Build history of the part. All positions in model axes, mm. A direction names the side the tool comes from. Round coordinates to 2 decimals unless told otherwise and drop trailing zeros. Loops run counter-clockwise (first coordinate to the right, second up) from the corner with the lowest first, then second, coordinate; pieces in that order, holes last. Notation, with made-up numbers: (23, 76) - (36, 76) arc R25 cw to (36, 95) - close; hole circle Ø4 at (-19, 89). An arc over 180 degrees is marked (long way). Put each result on its own line as item: value. Start each with the question number.
from build123d import *

# Parameters (mm, degrees)
SKETCH1_R               = 3.9
BOSS_EXTRUDE1_DEPTH     = 7
SKETCH2_R               = 6
BOSS_EXTRUDE2_DEPTH     = 1
SKETCH3_R               = 9.9
BOSS_EXTRUDE3_DEPTH     = 7
BOSS_EXTRUDE4_DEPTH     = 1
SKETCH5_R               = 1.6
CUT_EXTRUDE1_DEPTH      = 20.300518128
CUT_EXTRUDE2_DEPTH      = 20.300518128
CUT_EXTRUDE2_DEPTH_BACK = 5
SKETCH7_R               = 3.5
CHAMFER1_SIZE           = 1


with BuildPart() as part:
    # Sketch1 → Boss-Extrude1 (new body)
    with BuildSketch(Plane(origin=(0, 0, 0), x_dir=(1, 0, 0), z_dir=(0, 1, 0))):
        with Locations(Location((0, 0, 0), (0, 0, 270))):
            Circle(SKETCH1_R)
    extrude(amount=BOSS_EXTRUDE1_DEPTH)

    # Sketch2 → Boss-Extrude2 (add)
    with BuildSketch(Plane(origin=(0, 0, 0), x_dir=(-1, 0, 0), z_dir=(0, -1, 0))):
        with Locations(Location((0, 0, 0), (0, 0, 90))):
            Circle(SKETCH2_R)
    extrude(amount=BOSS_EXTRUDE2_DEPTH)

    # Sketch3 → Boss-Extrude3 (add)
    with BuildSketch(Plane(origin=(0, -1, 0), x_dir=(-1, 0, 0), z_dir=(0, -1, 0))):
        with Locations(Location((0, 2.5, 0), (0, 0, 90))):
            Circle(SKETCH3_R)
    extrude(amount=BOSS_EXTRUDE3_DEPTH)

    # Sketch4 → Boss-Extrude4 (add)
    with BuildSketch(Plane(origin=(0, -8, 0), x_dir=(-1, 0, 0), z_dir=(0, -1, 0))):
        with BuildLine():
            ThreePointArc((-11.736694594, 0), (0, -9.5), (11.736694594, 0))
            ThreePointArc((11.736694594, 0), (0, 9.5), (-11.736694594, 0))
        make_face()
    extrude(amount=BOSS_EXTRUDE4_DEPTH)

    # Sketch5 → Cut-Extrude1 (cut, through all)
    with BuildSketch(Plane(origin=(0, 0, 0), x_dir=(1, 0, 0), z_dir=(0, 1, 0))):
        with Locations(Location((5.5, 0, 0), (0, 0, 270))):
            Circle(SKETCH5_R)
        with Locations(Location((-5.5, 0, 0), (0, 0, 270))):
            Circle(SKETCH5_R)
    extrude(amount=-CUT_EXTRUDE1_DEPTH, mode=Mode.SUBTRACT)

    # Sketch7 → Cut-Extrude2 (cut, two sides: drawn at the far end of the back side and taken through both)
    with BuildSketch(Plane(origin=(0, 0, 0), x_dir=(1, 0, 0), z_dir=(0, 1, 0)).offset(-CUT_EXTRUDE2_DEPTH_BACK)):
        with Locations(Location((-5.5, 0, 0), (0, 0, 80.280132298))):
            Circle(SKETCH7_R)
        with Locations(Location((5.5, 0, 0), (0, 0, 99.719867702))):
            Circle(SKETCH7_R)
    extrude(amount=CUT_EXTRUDE2_DEPTH + CUT_EXTRUDE2_DEPTH_BACK, mode=Mode.SUBTRACT)

    # Chamfer1
    # the kernel refuses this chamfer: 1 mm, written as the material it takes off along each edge
    with BuildSketch(Plane(origin=(0, -1, -2.5), x_dir=(0, 0, -1), z_dir=(-1, 0, 0))) as chamfer1_piece_1:
        Polygon((9.9, CHAMFER1_SIZE), (9.9 - CHAMFER1_SIZE, 0), (9.9, 0), align=None)
    revolve(axis=Axis((0, -1, -2.5), (0, -1, 0)), mode=Mode.SUBTRACT)
    with BuildSketch(Plane(origin=(0, 7, 0), x_dir=(0.9996692397523004, 0, -0.025717913855091756), z_dir=(0.025717913855091756, 0, 0.9996692397523004))) as chamfer1_piece_2:
        Polygon((3.9 - CHAMFER1_SIZE, 0), (3.9, -CHAMFER1_SIZE), (3.9, 0), align=None)
    revolve(axis=Axis((0, 7, 0), (0, 1, 0)), revolution_arc=177.05261919, mode=Mode.SUBTRACT)
    with BuildSketch(Plane(origin=(0, 7, 0), x_dir=(0.9996692397523004, 0, 0.02571791385509249), z_dir=(0.02571791385509249, 0, -0.9996692397523004))) as chamfer1_piece_3:
        Polygon((3.9, CHAMFER1_SIZE), (3.9 - CHAMFER1_SIZE, 0), (3.9, 0), align=None)
    revolve(axis=Axis((0, 7, 0), (0, -1, 0)), revolution_arc=177.05261919, mode=Mode.SUBTRACT)


solid = part.part
Item 1: Drop flat-ended pins along their axis: pin 1 Ø3 at (x, z) = (-2.5, -7.5) entering from +Y; pin 2 Ø7.5 at (x, z) = (4, 1) entering from +Y; pin 3 Ø1.6 at (x, z) = (-1.5, 4.5) entering from +Y; pin 4 Ø6 at (y, z) = (-0.5, -8.5) entering from +X. Give the stop position or say it passes through.
Item 2: Slice it at B-B (y = -3). Give the cut face in (x, z), plus the area to 3 significant figures.
Item 3: Drill centre lines: probe 1 along X at (y, z) = (-4, -3); probe 2 along X at (y, z) = (-6.4, 0); probe 3 along Y at (x, z) = (-10.25, -3.5). Where is each one in solid material? Low to high. Write a range as [from, to].
Item 4: Slice it at A-A (x = 0). Give the cut face in (y, z).
Item 5: Which spindle directions (+Z, -Z, +X, -X, +Y, -Y) get a long thin tool onto all of the face, cutting with end or side? Do faces 1 (the cylindrical face through (-7.06, -6.97, -0.35)), 2 (the flat face through (0.1, 0, 4.3)), 3 (the flat face through (7, -5, -1)), 4 (the flat face through (1, -8, -10)), 5 (the flat face through (0, -1, -7)). Say none if no direction does.
Item 6: Slice it at C-C (y = 3.25). Give the cut face in (x, z), plus the area to 3 significant figures.
Computed values:
1. pin 1: stops at y = -1
1. pin 2: stops at y = 7
1. pin 3: stops at y = 0
1. pin 4: stops at x = 9.3
2. outline: circle Ø19.8 at (0, -2.5); hole circle Ø7 at (-5.5, 0); hole circle Ø7 at (5.5, 0)
2. area: 231 mm^2
3. probe 1: x = [-9.89, -7.3], [-3.7, 3.7], [7.3, 9.89]
3. probe 2: x = [-9.58, -7.1], [-3.9, 3.9], [7.1, 9.58]
3. probe 3: y = [-9, -8]
4. outline: (-9, -9.5) - (-8, -9.5) - (-8, -12.4) - (-2, -12.4) - (-1, -11.4) - (-1, -6) - (0, -6) - (0, -3.9) - (6, -3.9) - (7, -2.9) - (7, 2.9) - (6, 3.9) - (0, 3.9) - (0, 6) - (-1, 6) - (-1, 6.4) - (-2, 7.4) - (-8, 7.4) - (-8, 9.5) - (-9, 9.5) - close
5. face 1: +Y, -Y
5. face 2: +Z, +Y
5. face 3: +Y
5. face 4: -Z, -Y
5. face 5: -Z, +Y
6. outline: (-3.02, -2.47) arc R3.9 ccw to (3.02, -2.47) arc R3.5 cw to (3.02, 2.47) arc R3.9 ccw to (-3.02, 2.47) arc R3.5 cw to start
6. area: 34.9 mm^2
